The model under review builds one solid part; all positions refer to its coordinate system, in mm. A direction names the side the tool comes from. Give positions to 0.01 mm unless a question says otherwise; leave off trailing zeros. Order: outer loops, then holes, each group sorted by start corner. A loop starts at its lowest first (then second) coordinate and runs counter-clockwise, first axis right, second up.
```python
from build123d import *

# Parameters (mm, degrees)
SKETCH_1_W      = 17.6
SKETCH_1_H      = 5.8
EXTRUDE_1_DEPTH = 2.3
SKETCH_2_W      = 3.8
SKETCH_2_H      = 5.8
EXTRUDE_2_DEPTH = 9.7
SKETCH_5_R      = 0.225
EXTRUDE_3_DEPTH = 2


with BuildPart() as part:
    # 草图1 → 凸台-拉伸1 (new body)
    with BuildSketch(Plane(origin=(0, 0, 0), x_dir=(1, 0, 0), z_dir=(0, 1, 0))):
        Rectangle(SKETCH_1_W, SKETCH_1_H)
    extrude(amount=EXTRUDE_1_DEPTH)

    # 草图2 → 凸台-拉伸2 (add)
    with BuildSketch(Plane(origin=(0, 2.3, 0), x_dir=(1, 0, 0), z_dir=(0, 1, 0))):
        with Locations((-6.9, 0)):
            Rectangle(SKETCH_2_W, SKETCH_2_H)
        with Locations((6.9, 0)):
            Rectangle(SKETCH_2_W, SKETCH_2_H)
    extrude(amount=EXTRUDE_2_DEPTH)

    # 草图5 → 凸台-拉伸3 (add)
    with BuildSketch(Plane.XZ):
        with Locations(Location((-7.5, 1.27, 0), (0, 0, 90))):
            Circle(SKETCH_5_R)
        with Locations(Location((-7.5, -1.27, 0), (0, 0, 90))):
            Circle(SKETCH_5_R)
        with Locations(Location((7.5, 1.27, 0), (0, 0, 90))):
            Circle(SKETCH_5_R)
        with Locations(Location((7.5, -1.27, 0), (0, 0, 90))):
            Circle(SKETCH_5_R)
    extrude(amount=EXTRUDE_3_DEPTH)


solid = part.part
```
Item 1: Take a section at D-D (y = -0.5). Give the boundary of the cut face in (x, z) (3 decimals).
Values found:
outline: circle Ø0.45 at (-7.5, -1.27); circle Ø0.45 at (-7.5, 1.27); circle Ø0.45 at (7.5, -1.27); circle Ø0.45 at (7.5, 1.27)
Item 2: Take a section at B-B (z = 1.27). Give the boundary of the cut face in (x, y) (3 decimals), and give its area (3 significant figures).
Values found:
outline: (-8.8, 0) - (-7.725, 0) - (-7.725, -2) - (-7.275, -2) - (-7.275, 0) - (7.275, 0) - (7.275, -2) - (7.725, -2) - (7.725, 0) - (8.8, 0) - (8.8, 12) - (5, 12) - (5, 2.3) - (-5, 2.3) - (-5, 12) - (-8.8, 12) - close
area: 116 mm2
Item 3: For line 1 (X direction, y = 9.75, z = -2.1); line 2 (Y direction, x = 6.25, z = -0.85); line 3 (Y direction, x = 4.25, z = -0.2), list the stretches that pass through material, from the lowest coordinate up.
Values found:
line 1: x = -8.8 to -5, 5 to 8.8
line 2: y = 0 to 12
line 3: y = 0 to 2.3
Item 4: Clearance check with a flat-ended pin moving along its axis: pin 1 Ø3 at (x, z) = (4.5, 0.5) entering from -Y. State where the tip first meets the part, or that it passes through.
Values found:
pin 1: stops at y = 0
Item 5: For faces 4 (the flat face through (0, 2, 2.9)), 5 (the flat face through (-5, 7, 0)), list the 3-axis set-ups (+Z, -Z, +X, -X, +Y, -Y) from which the entire face can be reached by the end or side of a thin tool; tool diameter is ignored.
Values found:
face 4: +Z, +X, -X, +Y, -Y
face 5: +Z, -Z, +Y
Item 6: Take a section at A-A (y = 10.5). Give the boundary of the cut face in (x, z).
Values found:
outline: (-8.8, -2.9) - (-5, -2.9) - (-5, 2.9) - (-8.8, 2.9) - close; (5, -2.9) - (8.8, -2.9) - (8.8, 2.9) - (5, 2.9) - close
Item 7: Draft analysis for pull direction X (two halves, no side actions). For faces 1 (the flat face through (-8.8, 6, 0)), 2 (the flat face through (0, 2.3, 0)), 3 (the flat face through (7, 12, 0)), state which applies: released by +X, released by -X, zero draft, split by the parting line, or undercut.
Values found:
face 1: released by -X
face 2: undercut
face 3: zero draft
Item 8: Take a section at C-C (x = 7.5). Give the boundary of the cut face in (y, z) (3 decimals).
Values found:
outline: (-2, -1.495) - (0, -1.495) - (0, -2.9) - (12, -2.9) - (12, 2.9) - (0, 2.9) - (0, 1.495) - (-2, 1.495) - (-2, 1.045) - (0, 1.045) - (0, -1.045) - (-2, -1.045) - close
